```python
from build123d import *

# Parameters (mm, degrees)
SKETCH1_W           = 187
SKETCH1_H           = 158
SKETCH1_W_2         = 183
SKETCH1_H_2         = 154
BOSS_EXTRUDE1_DEPTH = 66
SKETCH2_W           = 187
SKETCH2_H           = 158
BOSS_EXTRUDE2_DEPTH = 2
FILLET1_R           = 10
FILLET2_R           = 10
SKETCH3_R           = 3
BOSS_EXTRUDE3_DEPTH = 32
SKETCH4_W           = 97
SKETCH4_H           = 40
CUT_EXTRUDE1_DEPTH  = 10
SKETCH5_R           = 1.5
CUT_EXTRUDE2_DEPTH  = 10
SKETCH6_R           = 8
SKETCH6_W           = 13
SKETCH6_H           = 19
CUT_EXTRUDE3_DEPTH  = 10
FILLET3_R           = 2


with BuildPart() as part:
    # Sketch1 → Boss-Extrude1 (new body)
    with BuildSketch(Plane.XY):
        Rectangle(SKETCH1_W, SKETCH1_H)
        Rectangle(SKETCH1_W_2, SKETCH1_H_2, mode=Mode.SUBTRACT)
    extrude(amount=BOSS_EXTRUDE1_DEPTH)

    # Sketch2 → Boss-Extrude2 (add)
    with BuildSketch(Plane(origin=(0, 0, 0), x_dir=(-1, 0, 0), z_dir=(0, 0, -1))):
        Rectangle(SKETCH2_W, SKETCH2_H)
    extrude(amount=BOSS_EXTRUDE2_DEPTH)

    # Fillet1
    fillet1_edges = [part.edges().sort_by_distance(p)[0] for p in [
        (91.5, -77, 33),
        (91.5, 77, 33),
        (-91.5, 77, 33),
        (-91.5, -77, 33),
    ]]
    fillet(fillet1_edges, radius=FILLET1_R)

    # Fillet2
    fillet2_edges = [part.edges().sort_by_distance(p)[0] for p in [
        (93.5, -79, 32),
        (-93.5, -79, 32),
        (-93.5, 79, 32),
        (93.5, 79, 32),
    ]]
    fillet(fillet2_edges, radius=FILLET2_R)

    # Sketch3 → Boss-Extrude3 (add)
    with BuildSketch(Plane.XY):
        with Locations((-65.5, 33)):
            Circle(SKETCH3_R)
        with Locations((65.5, 33)):
            Circle(SKETCH3_R)
        with Locations((65.5, -33)):
            Circle(SKETCH3_R)
        with Locations((-65.5, -33)):
            Circle(SKETCH3_R)
    extrude(amount=BOSS_EXTRUDE3_DEPTH)

    # Sketch4 → Cut-Extrude1 (cut)
    with BuildSketch(Plane.XZ.offset(79)):
        with Locations((-19, 34)):
            Rectangle(SKETCH4_W, SKETCH4_H)
    extrude(amount=-CUT_EXTRUDE1_DEPTH, mode=Mode.SUBTRACT)

    # Sketch5 → Cut-Extrude2 (cut)
    with BuildSketch(Plane.XZ.offset(79)):
        with Locations((-65.5, 61.5)):
            Circle(SKETCH5_R)
        with Locations((27.5, 61.5)):
            Circle(SKETCH5_R)
        with Locations((-65.5, 6.5)):
            Circle(SKETCH5_R)
        with Locations((27.5, 6.5)):
            Circle(SKETCH5_R)
    extrude(amount=-CUT_EXTRUDE2_DEPTH, mode=Mode.SUBTRACT)

    # Sketch6 → Cut-Extrude3 (cut)
    with BuildSketch(Plane.XZ.offset(79)):
        with Locations((53.5, 46)):
            Circle(SKETCH6_R)
        with Locations((53.5, 18)):
            Rectangle(SKETCH6_W, SKETCH6_H)
    extrude(amount=-CUT_EXTRUDE3_DEPTH, mode=Mode.SUBTRACT)

    # Fillet3
    fillet3_edges = [part.edges().sort_by_distance(p)[0] for p in [
        (29.5, -78, 54),
        (29.5, -78, 14),
        (-67.5, -78, 14),
        (-67.5, -78, 54),
        (60, -78, 27.5),
        (60, -78, 8.5),
        (47, -78, 8.5),
        (47, -78, 27.5),
    ]]
    fillet(fillet3_edges, radius=FILLET3_R)


solid = part.part
```
CAD build for the part. Positions are in the model's coordinates, mm. A direction names the side the tool comes from. Round coordinates to 2 decimals unless told otherwise and drop trailing zeros. Write each loop counter-clockwise with the first axis right and the second up, starting at its lowest first coordinate (ties: lowest second). Pieces come first, ordered by that corner, then holes.
Item 1: Drop flat-ended pins along their axis: pin 1 Ø5 at (x, y) = (-64, 31.5) entering from +Z; pin 2 Ø20 at (x, z) = (-1.5, 35) entering from -Y; pin 3 Ø2 at (y, z) = (-78.5, 42.5) entering from -X. Give the stop position or say it passes through.
Filled in:
pin 1: stops at z = 32
pin 2: stops at y = 77
pin 3: stops at x = -88.77
Item 2: Band-saw the part on A-A on z = 46. Write the cut outline in (x, y).
Filled in:
outline: (-93.5, -69) arc R10 ccw to (-83.5, -79) - (-67.5, -79) - (-67.5, -77) - (-81.5, -77) arc R10 cw to (-91.5, -67) - (-91.5, 67) arc R10 cw to (-81.5, 77) - (81.5, 77) arc R10 cw to (91.5, 67) - (91.5, -67) arc R10 cw to (81.5, -77) - (61.5, -77) - (61.5, -79) - (83.5, -79) arc R10 ccw to (93.5, -69) - (93.5, 69) arc R10 ccw to (83.5, 79) - (-83.5, 79) arc R10 ccw to (-93.5, 69) - close; (29.5, -79) - (45.5, -79) - (45.5, -77) - (29.5, -77) - close
Item 3: Band-saw the part on B-B on x = -16. Write the cut outline in (y, z), then the cut area to 3 significant figures.
Filled in:
outline: (-79, -2) - (79, -2) - (79, 66) - (77, 66) - (77, 0) - (-77, 0) - (-77, 14) - (-79, 14) - close; (-79, 54) - (-77, 54) - (-77, 66) - (-79, 66) - close
area: 500 mm2
Item 4: Band-saw the part on D-D on x = 65.5. Write the cut outline in (y, z).
Filled in:
outline: (-79, -2) - (79, -2) - (79, 66) - (77, 66) - (77, 0) - (36, 0) - (36, 32) - (30, 32) - (30, 0) - (-30, 0) - (-30, 32) - (-36, 32) - (-36, 0) - (-77, 0) - (-77, 66) - (-79, 66) - close
Item 5: Mould opens along X. For faces 4 (the flat face through (1, 79, 32)), 5 (the cylindrical face through (90.49, 76.15, 32.48)), 6 (the flat face through (91.5, -1, 33)) say: released by +X, released by -X, zero draft, split by the parting line, or undercut.
Filled in:
face 4: zero draft
face 5: released by +X
face 6: undercut
Item 6: Band-saw the part on C-C on z = 23. Write the cut outline in (x, y).
Filled in:
outline: (-93.5, -69) arc R10 ccw to (-83.5, -79) - (-67.5, -79) - (-67.5, -77) - (-81.5, -77) arc R10 cw to (-91.5, -67) - (-91.5, 67) arc R10 cw to (-81.5, 77) - (81.5, 77) arc R10 cw to (91.5, 67) - (91.5, -67) arc R10 cw to (81.5, -77) - (60, -77) - (60, -79) - (83.5, -79) arc R10 ccw to (93.5, -69) - (93.5, 69) arc R10 ccw to (83.5, 79) - (-83.5, 79) arc R10 ccw to (-93.5, 69) - close; circle Ø6 at (-65.5, -33); circle Ø6 at (-65.5, 33); (29.5, -79) - (47, -79) - (47, -77) - (29.5, -77) - close; circle Ø6 at (65.5, -33); circle Ø6 at (65.5, 33)
Item 7: Drill centre lines: L1, parallel to Z at x = 27.5, y = -78.5; L2, parallel to Z at x = 53.5, y = -78.5; L3, parallel to X at y = -40, z = 63.5. Where is each one in solid material? Low to high.
Filled in:
L1: z = -2 to 5, 8 to 14, 54 to 60, 63 to 66
L2: z = -2 to 8.5, 27.5 to 38, 54 to 66
L3: x = -93.5 to -91.5, 91.5 to 93.5
Item 8: Tool access for faces 1 (the cylindrical face through (52.459, -78.014, 53.932)), 2 (the cylindrical face through (88.49, 74.15, 33.46)), 3 (the flat face through (1, 1, -2)): list every direction of +Z, -Z, +X, -X, +Y, -Y with a clear straight run to the whole face (end or side of a thin tool).
Filled in:
face 1: -Y
face 2: +Z
face 3: -Z, +X, -X, +Y, -Y
